Read the model definition and answer for the solid it produces. Units are mm, in the model's axes. Face numbers are marked on the shaded views. A direction names the side the tool comes from. Coordinates: 2 decimals unless noted, no trailing zeros. Loops run counter-clockwise (first coordinate to the right, second up) from the corner with the lowest first, then second, coordinate; pieces in that order, holes last. Notation, with made-up numbers: (85.5, -18.75) - (114.5, -18.75) arc R37 ccw to (114.5, 17.25) - close; hole circle Ø1 at (66, 20.5). An arc over 180 degrees is marked (long way). One line per item, written item: value. Start each with the question number.
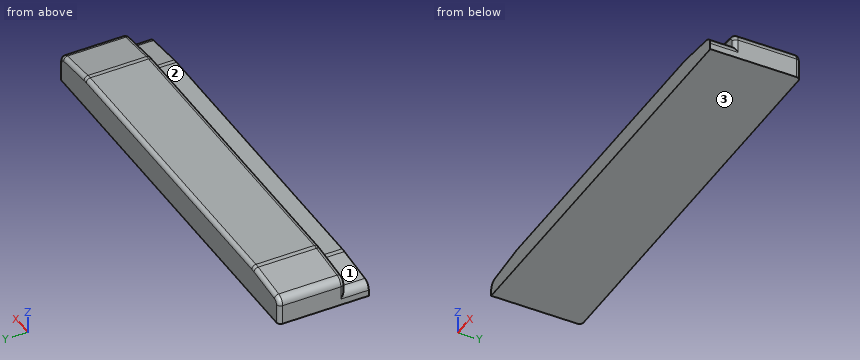
from build123d import *

# Parameters (mm, degrees)
BOSS_EXTRUDE1_DEPTH = 168.275
CUT_EXTRUDE1_DEPTH  = 44.45
FILLET1_R           = 15.24
FILLET2_R           = 76.2
FILLET3_R           = 7.62
FILLET4_R           = 7.62


with BuildPart() as part:
    # Sketch7 → Boss-Extrude1 (new body)
    with BuildSketch(Plane(origin=(0, 0, 0), x_dir=(1, 0, 0), z_dir=(0, 1, 0))):
        Polygon((0, 0), (762, 0), (762, -50.8), (673.1, -60.325), (88.9, -60.325), (0, -50.8), align=None)
    extrude(amount=BOSS_EXTRUDE1_DEPTH)

    # Sketch10 → Cut-Extrude1 (cut)
    with BuildSketch(Plane.XZ):
        Polygon((0, 50.8), (0, 25.4), (88.9, 34.925), (673.1, 34.925), (762, 25.4), (762, 50.8), (673.1, 60.325), (88.9, 60.325), align=None)
    extrude(amount=-CUT_EXTRUDE1_DEPTH, mode=Mode.SUBTRACT)

    # Fillet1
    fillet1_edges = [part.edges().sort_by_distance(p)[0] for p in [
        (762, 106.3625, 50.8),
        (0, 106.3625, 50.8),
        (762, 22.225, 25.4),
        (0, 22.225, 25.4),
    ]]
    fillet(fillet1_edges, radius=FILLET1_R)

    # Fillet2
    fillet2_edges = [part.edges().sort_by_distance(p)[0] for p in [
        (673.1, 106.3625, 60.325),
        (88.9, 106.3625, 60.325),
        (673.1, 22.225, 34.925),
        (88.9, 22.225, 34.925),
    ]]
    fillet(fillet2_edges, radius=FILLET2_R)

    # Fillet3
    fillet3_edges = [part.edges().sort_by_distance(p)[0] for p in [
        (762, 168.275, 18.552816133),
        (0, 168.275, 18.552816133),
        (49.234552732, 168.275, 56.07513065),
        (3.904199904, 168.275, 47.291761863),
        (758.095800096, 168.275, 47.291761863),
        (712.765447268, 168.275, 56.07513065),
        (381, 168.275, 60.325),
        (88.905795265, 168.275, 60.216512154),
        (673.094204735, 168.275, 60.216512154),
    ]]
    fillet(fillet3_edges, radius=FILLET3_R)

    # Fillet4
    fillet4_edges = [part.edges().sort_by_distance(p)[0] for p in [
        (762, 44.45, 18.552816133),
        (0, 44.45, 18.552816133),
        (712.765447268, 44.45, 56.07513065),
        (3.904199904, 44.45, 47.291761863),
        (758.095800096, 44.45, 47.291761863),
        (381, 44.45, 60.325),
        (49.234552732, 44.45, 56.07513065),
        (88.905795265, 44.45, 60.216512154),
        (673.094204735, 44.45, 60.216512154),
    ]]
    fillet(fillet4_edges, radius=FILLET4_R)


solid = part.part
1) A flat-ended cylindrical pin translates along its axis: P1, Ø12, axis at y = 60, z = 49.5, coming from the +X side. Find the tip coordinate at first contact, or state that the pin passes through.
2) For the marked faces 1, 2 and 3, determine the directions among +Z, -Z, +X, -X, +Y, -Y from which every point of the face is accessible in a straight line to the end or side of a thin tool.
3) Section C-C, the plane y = 32 is taken. Determine the outline of the cut face in (x, z) (1 decimal).
4) Section B-B, the plane y = 134 is taken. Determine the outline of the cut face in (x, z) (1 decimal), and give its area (3 significant figures).
5) Straight lines are drawn through the part: L1, parallel to Z at x = 668, y = 8.5 (3 decimals); L2, parallel to Y at x = 42, z = 39.5 (3 decimals); L3, parallel to X at y = 136, z = 38. For each, find the intervals that lie inside material, in ascending order.
6) Section A-A, the plane x = 417 is taken. Determine the outline of the cut face in (y, z) (3 decimals).
Answer below:
1. P1: x = 760.59
2. face 1: +Z, -X, -Y
2. face 2: +Z, +X, -X, -Y
2. face 3: -Z, +X, -X, +Y, -Y
3. outline: (0, 0) - (762, 0) - (762, 11.7) arc R15.2 ccw to (748.4, 26.9) - (677.1, 34.5) arc R76.2 ccw to (669, 34.9) - (93, 34.9) arc R76.2 ccw to (84.9, 34.5) - (13.6, 26.9) arc R15.2 ccw to (0, 11.7) - close
4. outline: (0, 0) - (762, 0) - (762, 37.1) arc R15.2 ccw to (748.4, 52.3) - (677.1, 59.9) arc R76.2 ccw to (669, 60.3) - (93, 60.3) arc R76.2 ccw to (84.9, 59.9) - (13.6, 52.3) arc R15.2 ccw to (0, 37.1) - close
4. area: 45,000 mm2
5. L1: 0 to 34.925
5. L2: 44.45 to 168.275
5. L3: 0.03 to 761.97
6. outline: (0, 0) - (168.275, 0) - (168.275, 52.705) arc R7.62 ccw to (160.655, 60.325) - (52.07, 60.325) arc R7.62 ccw to (44.45, 52.705) - (44.45, 34.925) - (0, 34.925) - close
